Check sheet for the drawn part. Datum: minimum x, y, z corner. Units: mm. Give positions to 0.01 mm unless a question says otherwise; leave off trailing zeros. Loops run counter-clockwise (first coordinate to the right, second up) from the corner with the lowest first, then second, coordinate; pieces in that order, holes last. Notation, with made-up numbers: (29.5, 44) - (80.5, 44) arc R20 ccw to (80.5, 78) - close; hole circle Ø9 at (5, 78.25). An arc over 180 degrees is marked (long way). Use one line per item in the form item = value.
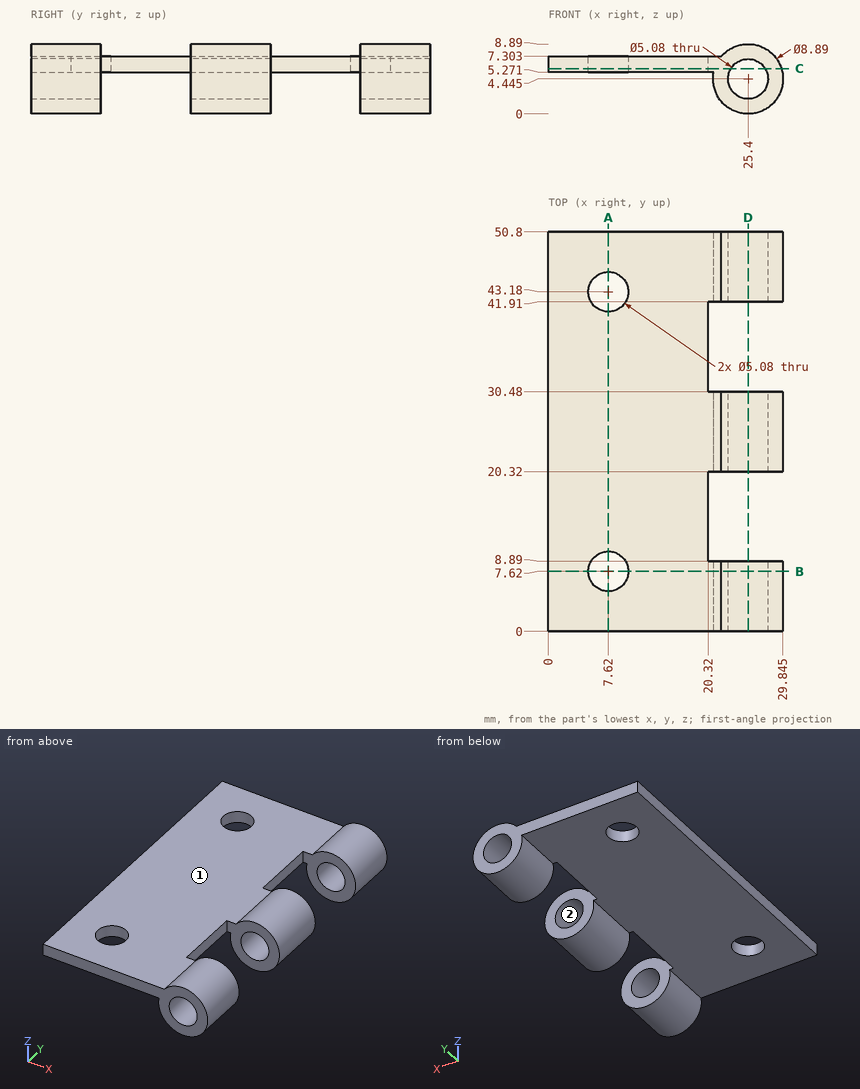
1. Draft check along Z on the marked faces 1 and 2. Enter one of: released by +Z, released by -Z, zero draft, split by the parting line, or undercut.
Result set:
face_1 = released by +Z
face_2 = undercut
2. Section check D-D, the plane x = 25.4. Record the cut outline in (y, z) (1 decimal).
Result set:
outline = (0, 0) - (8.9, 0) - (8.9, 1.9) - (0, 1.9) - close; (0, 7) - (8.9, 7) - (8.9, 8.9) - (0, 8.9) - close; (20.3, 0) - (30.5, 0) - (30.5, 1.9) - (20.3, 1.9) - close; (20.3, 7) - (30.5, 7) - (30.5, 8.9) - (20.3, 8.9) - close; (41.9, 0) - (50.8, 0) - (50.8, 1.9) - (41.9, 1.9) - close; (41.9, 7) - (50.8, 7) - (50.8, 8.9) - (41.9, 8.9) - close
3. Depth check by flat-ended pin: pin 1 Ø8 at (x, y) = (12.5, 13.5) entering from +Z; pin 2 Ø5 at (x, y) = (13.5, 13) entering from -Z; pin 3 Ø0.6 at (y, z) = (15.5, 6) entering from +X. Enter the tip coordinate at first touch or a pass-through.
Result set:
pin_1 = 7.3
pin_2 = 5.27
pin_3 = 20.32
4. Section check C-C, the plane z = 5.75. Record the cut outline in (x, y).
Result set:
outline = (0, 0) - (23.22, 0) - (23.22, 8.89) - (20.32, 8.89) - (20.32, 20.32) - (23.22, 20.32) - (23.22, 30.48) - (20.32, 30.48) - (20.32, 41.91) - (23.22, 41.91) - (23.22, 50.8) - (0, 50.8) - close; (27.58, 0) - (29.65, 0) - (29.65, 8.89) - (27.58, 8.89) - close; (27.58, 20.32) - (29.65, 20.32) - (29.65, 30.48) - (27.58, 30.48) - close; (27.58, 41.91) - (29.65, 41.91) - (29.65, 50.8) - (27.58, 50.8) - close; hole circle Ø5.08 at (7.62, 7.62); hole circle Ø5.08 at (7.62, 43.18)
5. Section check A-A, the plane x = 7.62. Record the cut outline in (y, z).
Result set:
outline = (0, 5.27) - (5.08, 5.27) - (5.08, 7.3) - (0, 7.3) - close; (10.16, 5.27) - (40.64, 5.27) - (40.64, 7.3) - (10.16, 7.3) - close; (45.72, 5.27) - (50.8, 5.27) - (50.8, 7.3) - (45.72, 7.3) - close
6. Scan lines: probe 1 along Y at (x, z) = (7.62, 6.2); probe 2 along Y at (x, z) = (22.75, 5.5); probe 3 along Z at (x, y) = (17, 15). Record each from-to range of solid material in increasing order.
Result set:
probe_1 = 0 to 5.08, 10.16 to 40.64, 45.72 to 50.8
probe_2 = 0 to 8.89, 20.32 to 30.48, 41.91 to 50.8
probe_3 = 5.27 to 7.3
7. Section check B-B, the plane y = 7.62. Record the cut outline in (x, z) (1 decimal).
Result set:
outline = (0, 5.3) - (5.1, 5.3) - (5.1, 7.3) - (0, 7.3) - close; (10.2, 5.3) - (21, 5.3) arc R4.4 ccw (long way) to (22, 7.3) - (10.2, 7.3) - close; hole circle Ø5.1 at (25.4, 4.4)
